Verification items for the finished model (mm, model axes). Face numbers are marked on the shaded views. A direction names the side the tool comes from. Round coordinates to 2 decimals unless told otherwise and drop trailing zeros. Write each loop counter-clockwise with the first axis right and the second up, starting at its lowest first coordinate (ties: lowest second). Pieces come first, ordered by that corner, then holes.
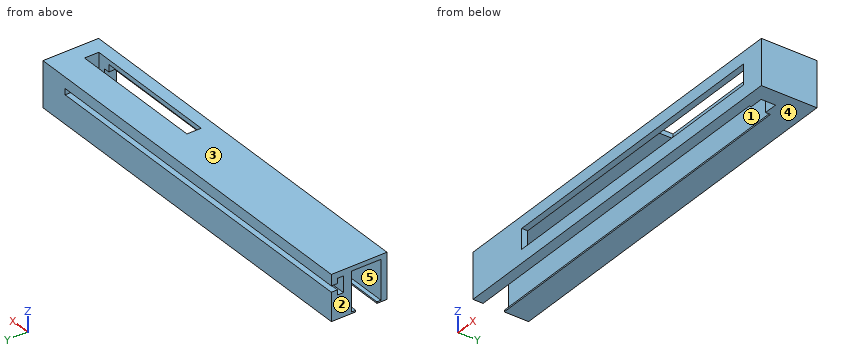
from build123d import *

# Parameters (mm, degrees)
F0_W     = 130
F0_H     = 18.43
F0_W_2   = 46.176888
F0_H_2   = 4.73
F1_DEPTH = 15
F2_W     = 7
F2_H     = 0.5
F3_DEPTH = 120
F4_W     = 100
F4_H     = 6.68
F5_DEPTH = 5


with BuildPart() as f1:
    # F0 (on Top) → F1 (new body)
    with BuildSketch(Plane.XY):
        Rectangle(F0_W, F0_H)
        with Locations((36.411556, -2.85)):
            Rectangle(F0_W_2, F0_H_2, mode=Mode.SUBTRACT)
    extrude(amount=F1_DEPTH)

    # F2 (on face) → F3 (cut)
    with BuildSketch(Plane(origin=(-65, 0, 0), x_dir=(0, -1, 0), z_dir=(-1, 0, 0))):
        Polygon((7.215, 13.5), (-2.485, 13.5), (-2.485, 0.5), (-1.135, 0.5), (5.865, 0.5), (7.215, 0.5), align=None)
        with Locations((2.365, 0.25)):
            Rectangle(F2_W, F2_H)
        Polygon((-7.215, 11.35), (-9.215, 11.35), (-9.215, 9.35), (-7.215, 9.35), (-7.215, 7.7), (-5.215, 7.7), (-5.215, 13), (-7.215, 13), align=None)
    extrude(amount=-F3_DEPTH, mode=Mode.SUBTRACT)

    # F4 (on face) → F5 (cut)
    with BuildSketch(Plane.XZ.offset(9.215)):
        with Locations((6.941007, 7.75)):
            Rectangle(F4_W, F4_H)
    extrude(amount=-F5_DEPTH, mode=Mode.SUBTRACT)


solid = f1.part
Q1. Sectioned sample at C-C (y = -3.25). Enter the section's corners in (x, z), plus the area to 3 significant figures.
Recorded:
outline: (-65, 13.5) - (13.32, 13.5) - (13.32, 15) - (-65, 15) - close; (59.5, 0) - (65, 0) - (65, 15) - (59.5, 15) - close
area: 200 mm2
Q2. Sectioned sample at D-D (x = -45). Enter the section's corners in (y, z) (3 decimals).
Recorded:
outline: (-9.215, 0) - (-5.865, 0) - (-5.865, 0.5) - (-7.215, 0.5) - (-7.215, 13.5) - (2.485, 13.5) - (2.485, 0.5) - (1.135, 0.5) - (1.135, 0) - (9.215, 0) - (9.215, 9.35) - (7.215, 9.35) - (7.215, 7.7) - (5.215, 7.7) - (5.215, 13) - (7.215, 13) - (7.215, 11.35) - (9.215, 11.35) - (9.215, 15) - (-9.215, 15) - close
Q3. Sectioned sample at A-A (x = -24). Enter the section's corners in (y, z) (3 decimals).
Recorded:
outline: (-9.215, 0) - (-5.865, 0) - (-5.865, 0.5) - (-7.215, 0.5) - (-7.215, 4.41) - (-9.215, 4.41) - close; (-9.215, 11.09) - (-7.215, 11.09) - (-7.215, 13.5) - (2.485, 13.5) - (2.485, 0.5) - (1.135, 0.5) - (1.135, 0) - (9.215, 0) - (9.215, 9.35) - (7.215, 9.35) - (7.215, 7.7) - (5.215, 7.7) - (5.215, 13) - (7.215, 13) - (7.215, 11.35) - (9.215, 11.35) - (9.215, 15) - (-9.215, 15) - close
Q4. Release check for a two-part mould opening along Z. For the marked faces 3, 4 and 5 record: released by +Z, released by -Z, zero draft, split by the parting line, or undercut.
Recorded:
face 3: released by +Z
face 4: released by -Z
face 5: undercut
Q5. Depth check by flat-ended pin: P1, Ø0.5, axis at x = 4, z = 8.5, coming from the -Y side (3 decimals); P2, Ø2, axis at y = -6, z = 2.5, coming from the -X side; P3, Ø4, axis at x = 2.5, y = -1.5, coming from the -Z side; P4, Ø2, axis at x = 25, y = -2, coming from the +Z side. Enter the tip coordinate at first touch or a pass-through.
Recorded:
P1: stops at y = 2.485
P2: stops at x = 55
P3: stops at z = 13.5
P4: passes through
Q6. Tool access check on the marked faces 1 and 2. Record the directions out of +Z, -Z, +X, -X, +Y, -Y that give a thin tool (end or side, any length) a straight path to the whole face; none if there is none.
Recorded:
face 1: -X
face 2: +Z, -Z, -X, +Y, -Y
Q7. Material ranges on line 1 along Y through (x, z) = (-47, 12) (3 decimals); line 2 along Z through (x, y) = (51, 8.75); line 3 along Z through (x, y) = (17, 1.5), recorded low to high.
Recorded:
line 1: y = -9.215 to -7.215, 2.485 to 5.215, 7.215 to 9.215
line 2: z = 0 to 9.35, 11.35 to 15
line 3: z = 0 to 0.5, 13.5 to 15
Q8. Sectioned sample at B-B (z = 6.25). Enter the section's corners in (x, y) (3 decimals).
Recorded:
outline: (-65, -9.215) - (-43.059, -9.215) - (-43.059, -7.215) - (-65, -7.215) - close; (-65, 2.485) - (55, 2.485) - (55, -0.485) - (59.5, -0.485) - (59.5, -5.215) - (56.941, -5.215) - (56.941, -9.215) - (65, -9.215) - (65, 9.215) - (-65, 9.215) - close
